Check sheet for the modelled part. Datum: model origin and axes. Units: mm. Give positions to 0.01 mm unless a question says otherwise; leave off trailing zeros. Order: outer loops, then holes, each group sorted by start corner. A loop starts at its lowest first (then second) coordinate and runs counter-clockwise, first axis right, second up.
```python
from build123d import *

# Parameters (mm, degrees)
SKETCH1_R           = 2.5
SKETCH1_R_2         = 0.75
BOSS_EXTRUDE1_DEPTH = 3
BOSS_EXTRUDE2_START = -6
SKETCH2_R           = 3
SKETCH2_R_2         = 2.5
BOSS_EXTRUDE2_DEPTH = 3


with BuildPart() as part:
    # Sketch1 → Boss-Extrude1 (new body)
    with BuildSketch(Plane(origin=(0, 0, 0), x_dir=(1, 0, 0), z_dir=(0, 1, 0))):
        with BuildLine():
            Line((0.278745645, 3.990275788), (28.839372822, 1.995137894))
            ThreePointArc((28.839372822, 1.995137894), (30.7, 0), (28.839372822, -1.995137894))
            Line((28.839372822, -1.995137894), (0.278745645, -3.990275788))
            ThreePointArc((0.278745645, -3.990275788), (-4, 0), (0.278745645, 3.990275788))
        make_face()
        with Locations(Location((0, 0, 0), (0, 0, 270))):
            Circle(SKETCH1_R, mode=Mode.SUBTRACT)
        with Locations(Location((28.7, 0, 0), (0, 0, 270))):
            Circle(SKETCH1_R_2, mode=Mode.SUBTRACT)
    extrude(amount=BOSS_EXTRUDE1_DEPTH)

    # Sketch2 → Boss-Extrude2 (add)
    with BuildSketch(Plane(origin=(0, 3, 0), x_dir=(1, 0, 0), z_dir=(0, 1, 0)).offset(BOSS_EXTRUDE2_START)):
        with Locations(Location((0, 0, 0), (0, 0, 270))):
            Circle(SKETCH2_R)
        with Locations(Location((0, 0, 0), (0, 0, 270))):
            Circle(SKETCH2_R_2, mode=Mode.SUBTRACT)
    extrude(amount=BOSS_EXTRUDE2_DEPTH)


solid = part.part
```
(1) Sectioned sample at A-A (z = 0). Enter the section's corners in (x, y).
(2) Thickness scan on L1, parallel to X at y = 1.7, z = 0; L2, parallel to X at y = -0.5, z = 0; L3, parallel to Y at x = 24, z = -0.75. Record the ranges inside material, lowest first.
(3) Sectioned sample at B-B (y = 1.9). Enter the section's corners in (x, z).
(4) Sectioned sample at C-C (x = 1.5). Enter the section's corners in (y, z), plus the area to 3 significant figures.
(5) Release check for a two-part mould opening along Z. For faces 1 (the face through (29.444, 1.479, -0.098)), 2 (the face through (0.9, -1.52, 2.86)), 3 (the face through (14, 3, 0)) record: released by +Z, released by -Z, zero draft, split by the parting line, or undercut.
(6) Sectioned sample at D-D (y = -0.75). Enter the section's corners in (x, z).
(7) Go/stop test with flat-tipped pins: P1, Ø1, axis at x = 4.5, y = 2.5, coming from the -Z side; P2, Ø1, axis at x = 3, y = 1, coming from the -Z side; P3, Ø3, axis at x = 0, z = 0, coming from the -Y side; P4, Ø2, axis at x = 12.5, z = 1, coming from the -Y side. Record where each tip stops, or that it passes through.
Values follow:
1. outline: (-4, 0) - (-3, 0) - (-3, -3) - (-2.5, -3) - (-2.5, 3) - (-4, 3) - close; (2.5, -3) - (3, -3) - (3, 0) - (27.95, 0) - (27.95, 3) - (2.5, 3) - close; (29.45, 0) - (30.7, 0) - (30.7, 3) - (29.45, 3) - close
2. L1: x = -4 to -2.5, 2.5 to 27.95, 29.45 to 30.7
2. L2: x = -3 to -2.5, 2.5 to 3
2. L3: y = 0 to 3
3. outline: (0.28, -3.99) - (28.84, -2) arc R2 ccw to (28.84, 2) - (0.28, 3.99) arc R4 ccw (long way) to start; hole circle Ø5 at (0, 0); hole circle Ø1.5 at (28.7, 0)
4. outline: (-3, -2.6) - (0, -2.6) - (0, -3.9) - (3, -3.9) - (3, -2) - (-3, -2) - close; (-3, 2) - (3, 2) - (3, 3.9) - (0, 3.9) - (0, 2.6) - (-3, 2.6) - close
4. area: 15.0 mm2
5. face 1: undercut
5. face 2: split by the parting line
5. face 3: zero draft
6. outline: circle Ø6 at (0, 0); hole circle Ø5 at (0, 0)
7. P1: stops at z = -3.73
7. P2: stops at z = -3.84
7. P3: passes through
7. P4: stops at y = 0
